Design review of the part shown in the three views and the two pictorial views. Dimensions are in mm from the part's minimum x, y and z. A direction names the side the tool comes from. Give positions to 0.01 mm unless a question says otherwise; leave off trailing zeros.
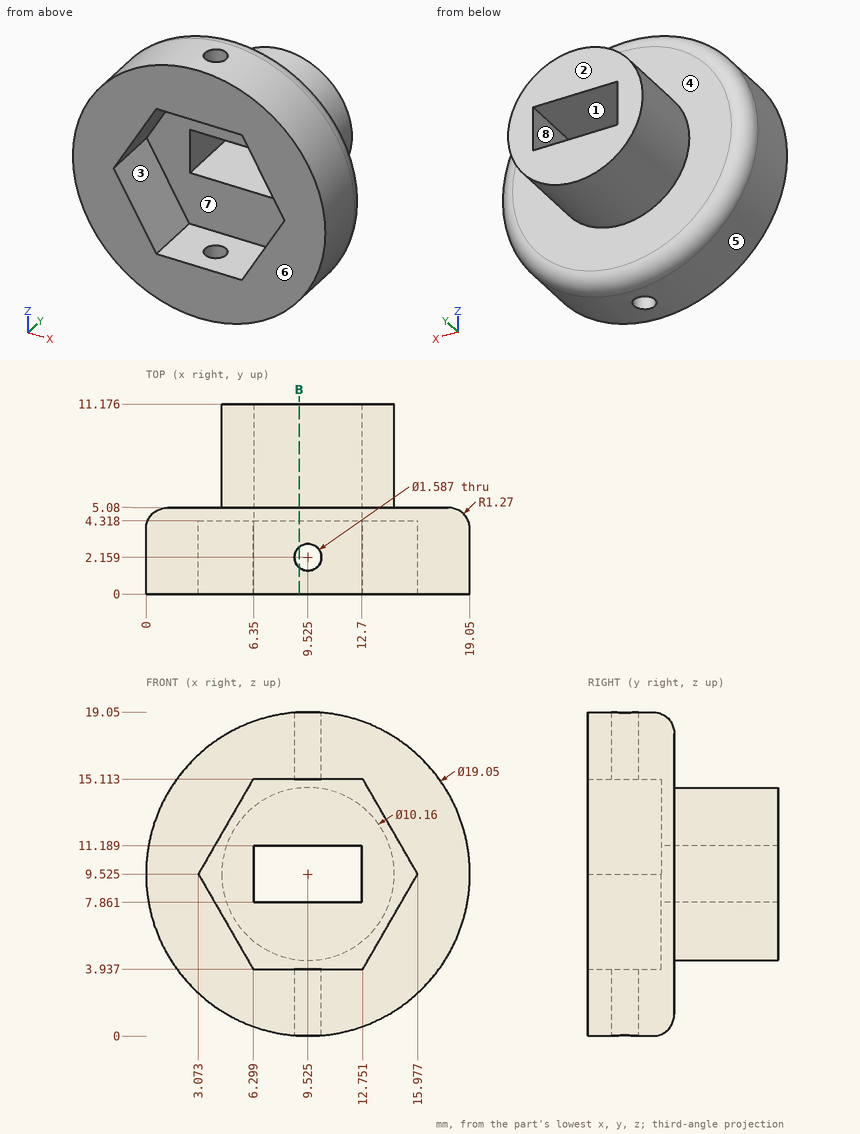
(1) Tool access review of the marked faces 1, 2, 3 and 4: name each direction out of +Z, -Z, +X, -X, +Y, -Y from which nothing blocks a thin tool from reaching the whole face with its end or side.
Resolved:
face 1: +Y, -Y
face 2: +Z, -Z, +X, -X, +Y
face 3: -Y
face 4: +Y
(2) Mouldability with a two-part tool opening along X and no side actions: class the marked faces 5, 6, 7 and 8 as pulls with the +X half, pulls with the -X half, needs draft (parallel to the pull), parting line crosses it, or undercut.
Resolved:
face 5: parting line crosses it
face 6: needs draft
face 7: undercut
face 8: undercut
(3) To check wall thickness, follow L1, parallel to Z at x = 9.75, y = 10; L2, parallel to X at y = 10.25, z = 10.5; L3, parallel to X at y = 8, z = 9. State the ranges of each line that lie inside material, in increasing order.
Resolved:
L1: z = 4.45 to 7.86, 11.19 to 14.6
L2: x = 4.54 to 6.35, 12.7 to 14.51
L3: x = 4.47 to 6.35, 12.7 to 14.58
(4) Clearance check with flat-ended pins moving along their axes: P1, Ø5, axis at x = 9.5, y = 8.5, coming from the -Z side (1 decimal); P2, Ø2, axis at x = 9.525, y = 2.159, coming from the -Z side; P3, Ø1.3, axis at x = 9.525, y = 2.159, coming from the +Z side; P4, Ø2.5, axis at y = 7, z = 10.5, coming from the -X side (1 decimal). State where each tip first meets the part, or that it passes through.
Resolved:
P1: stops at z = 4.4
P2: stops at z = 0
P3: passes through
P4: stops at x = 4.4
(5) Consider section B-B, the plane x = 9. Give the number of separate pieces and of enclosed holes in the cut face.
Resolved:
separate pieces: 4
enclosed holes: 0
